The figure shows three views and two pictorial views of one solid part (mm, origin at its lowest corner). Answer the questions. Round coordinates to 2 decimals unless told otherwise and drop trailing zeros. Order: outer loops, then holes, each group sorted by start corner. A loop starts at its lowest first (then second) coordinate and runs counter-clockwise, first axis right, second up. Notation, with made-up numbers: (-12.5, 88.25) -> (44.5, 88.25) arc R25 ccw to (44.5, 103.25) -> close; hole circle Ø3 at (59, -40). An arc over 180 degrees is marked (long way). One line per item, written item: value. Start each with the question number.
1. Section A-A (y = 28) is taken. Give the vertices of the cut face in (x, z) (3 decimals), then the cut area to 3 significant figures.
2. Consider line 1 (Z direction, x = 2.4, y = 68.5); line 2 (Y direction, x = 1.85, z = 75) (3 decimals). Determine where each line is inside the solid, lowest interval first.
3. Flat-ended cylindrical pins translate along their axes: pin 1 Ø1.6 at (x, y) = (1.5, 29) entering from +Z; pin 2 Ø1 at (x, z) = (1, 97.5) entering from -Y; pin 3 Ø1 at (x, z) = (1, 74) entering from -Y (3 decimals). Find the tip coordinate at first contact, or state that the pin passes through.
4. Section B-B (z = 73) is taken. Give the vertices of the cut face in (x, y) (3 decimals), then the cut area to 3 significant figures.
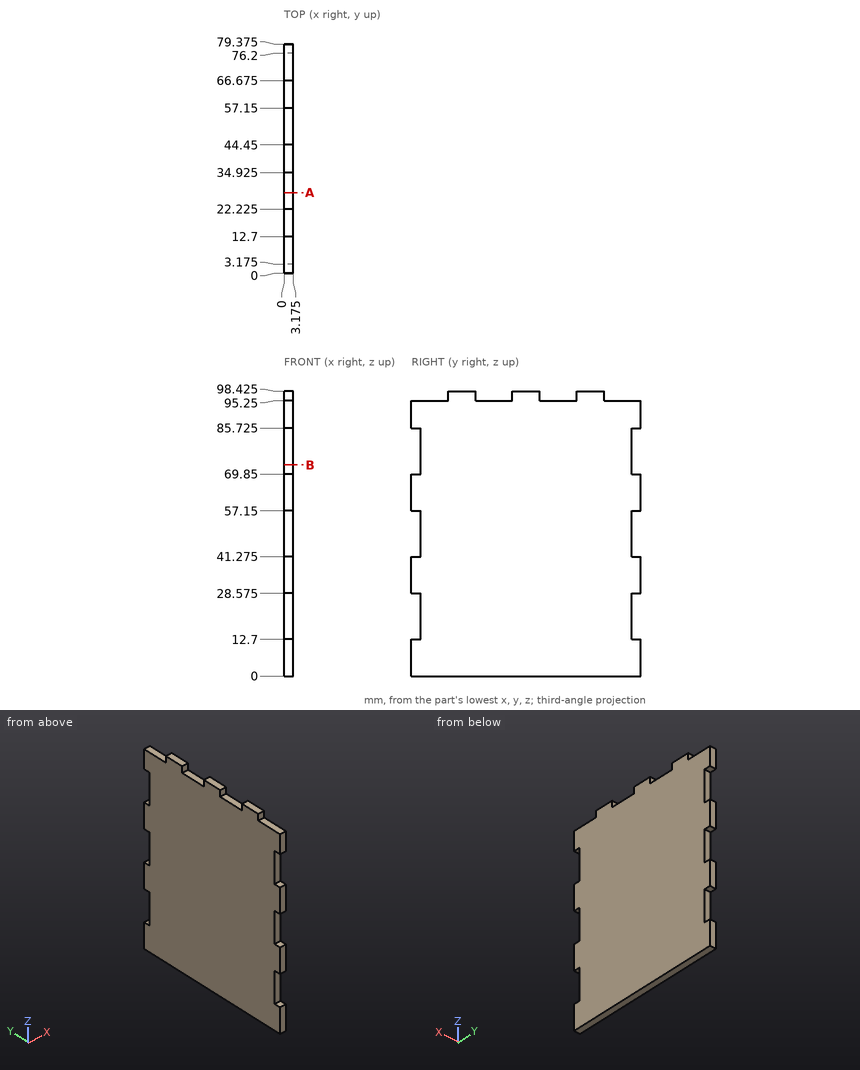
Answer:
1. outline: (0, 0) -> (3.175, 0) -> (3.175, 95.25) -> (0, 95.25) -> close
1. area: 302 mm^2
2. line 1: 0 to 95.25
2. line 2: 3.175 to 76.2
3. pin 1: z = 95.25
3. pin 2: y = 12.7
3. pin 3: y = 3.175
4. outline: (0, 3.175) -> (3.175, 3.175) -> (3.175, 76.2) -> (0, 76.2) -> close
4. area: 232 mm^2
